Design review of the part built by this model. Coordinates are the model's own, in mm. A direction names the side the tool comes from. Give positions to 0.01 mm unless a question says otherwise; leave off trailing zeros. Write each loop counter-clockwise with the first axis right and the second up, starting at its lowest first coordinate (ties: lowest second). Pieces come first, ordered by that corner, then holes. Notation, with made-up numbers: M -39,-32.5 L -9,-32.5 A22 cw -9,-14.5 Z; hole C 87,66.5 d6. An arc over 180 degrees is marked long. Answer in a Markdown table with one row per item.
```python
from build123d import *

# Parameters (mm, degrees)
SKETCH2_R          = 6.35
CUT_EXTRUDE1_DEPTH = 76.201267443
CIRPATTERN1_COUNT  = 6


with BuildPart() as part:
    # Sketch1 → Revolve1 (revolve)
    with BuildSketch(Plane(origin=(0, 0, 0), x_dir=(0, 0, -1), z_dir=(1, 0, 0)), mode=Mode.PRIVATE) as revolve1_sk:
        Polygon((19.05, 9.525), (-19.05, 9.525), (-19.05, 15.875), (-3.175, 19.05), (-3.175, 44.45), (-15.875, 47.625), (-15.875, 50.8), (15.875, 50.8), (15.875, 47.625), (3.175, 44.45), (3.175, 19.05), (19.05, 15.875), align=None)
    revolve(revolve1_sk.sketch.rotate(Axis((0, 0, 37.30886104), (0, 0, -1)), 90), axis=Axis((0, 0, 37.30886104), (0, 0, -1)))

    # Sketch2 → Cut-Extrude1 (cut, through all)
    with BuildSketch(Plane.XY.offset(3.175)):
        with Locations((0, 31.75)):
            Circle(SKETCH2_R)
    cut_extrude1 = extrude(amount=-CUT_EXTRUDE1_DEPTH, mode=Mode.SUBTRACT)

    # CirPattern1: Cut-Extrude1 ×6 about axis
    cirpattern1_axis = Axis((0, 0, 0), (0, 0, 1))
    for i in range(1, CIRPATTERN1_COUNT):
        add(cut_extrude1.rotate(cirpattern1_axis, i * 360 / CIRPATTERN1_COUNT), mode=Mode.SUBTRACT)


solid = part.part
```
1) For faces 5 (the face through (21.44, 13.97, 0.04)), 6 (the face through (9, 19, -3.175)), list the 3-axis set-ups (+Z, -Z, +X, -X, +Y, -Y) from which the entire face can be reached by the end or side of a thin tool; tool diameter is ignored.
Geometry says:
| item | result |
|---|---|
| face 5 | +Z, -Z |
| face 6 | -Z |
2) Add section A-A (y = 0). Write out the cut boundary in (x, z) (3 decimals).
Geometry says:
| item | result |
|---|---|
| outline | M -50.8,-15.875 L -47.625,-15.875 L -44.45,-3.175 L -19.05,-3.175 L -15.875,-19.05 L -9.525,-19.05 L -9.525,19.05 L -15.875,19.05 L -19.05,3.175 L -44.45,3.175 L -47.625,15.875 L -50.8,15.875 Z; M 9.525,-19.05 L 15.875,-19.05 L 19.05,-3.175 L 44.45,-3.175 L 47.625,-15.875 L 50.8,-15.875 L 50.8,15.875 L 47.625,15.875 L 44.45,3.175 L 19.05,3.175 L 15.875,19.05 L 9.525,19.05 Z |
3) Add section B-B (z = 6). Count the separate pieces of the cut face and the enclosed holes in it, and give its area (3 significant figures).
Geometry says:
| item | result |
|---|---|
| separate pieces | 2 |
| enclosed holes | 2 |
| area | 2,490 mm^2 |
4) To check wall thickness, follow probe 1 along Y at (x, z) = (0, 0.25) (3 decimals); probe 2 along X at (y, z) = (-15, 9.5); probe 3 along X at (y, z) = (-8, -5). State the ranges of each line that lie inside material, in increasing order. Write a range as [from, to].
Geometry says:
| item | result |
|---|---|
| probe 1 | [-50.8, -38.1], [-25.4, -9.525], [9.525, 25.4], [38.1, 50.8] |
| probe 2 | [-48.53, -43.52], [-9.56, 9.56], [43.52, 48.53] |
| probe 3 | [-50.17, -44.19], [-16.89, -5.17], [5.17, 16.89], [44.19, 50.17] |
5) Insertion check: P1, Ø12, axis at x = -9.5, z = -10, coming from the -Y side; P2, Ø5, axis at y = 9, z = -7, coming from the -X side; P3, Ø20.5, axis at x = -27.5, y = 15.88, coming from the +Z side (3 decimals); P4, Ø17, axis at x = 0, y = 0, coming from the -Z side. Each pin has a flat end and moves straight along its axis. Give the tip position at first contact, or say it passes through.
Geometry says:
| item | result |
|---|---|
| P1 | y = -50.68 |
| P2 | x = -50.38 |
| P3 | z = 3.175 |
| P4 | through |
6) The part is to be moulded in two halves that separate along X. For faces 1 (the face through (-9, 19, 3.175)), 2 (the face through (-40.313, 30.911, -0.222)), 3 (the face through (-15.3, -45.4, -15.875)), 4 (the face through (-9.669, 43.543, -3.792)), say which applies: released by +X, released by -X, zero draft, split by the parting line, or undercut.
Geometry says:
| item | result |
|---|---|
| face 1 | undercut |
| face 2 | split by the parting line |
| face 3 | zero draft |
| face 4 | undercut |
